Work out the finished part from the listing and answer in its coordinate system (mm). A direction names the side the tool comes from. Give positions to 0.01 mm unless a question says otherwise; leave off trailing zeros. Order: outer loops, then holes, each group sorted by start corner. A loop starts at its lowest first (then second) coordinate and runs counter-clockwise, first axis right, second up. Notation, with made-up numbers: (42.5, 66.5) -> (78.5, 66.5) arc R32 ccw to (78.5, 99.5) -> close; hole circle Ø9 at (84.25, 65.5). An arc over 180 degrees is marked (long way). Answer as CSV lines item,"result". Start each with the question number.
1. A cutting plane is placed at C-C (y = -28). Give the vertices of the cut face in (x, z).
2. Flat-ended cylindrical pins translate along their axes: pin 1 (1.9 mm diameter, centred on x = 19, z = 4, fed in from +Y); pin 2 (1.5 mm diameter, centred on x = -9, z = 1, fed in from +Y); pin 3 (1.9 mm diameter, centred on x = 18, z = 2, fed in from +Y); pin 4 (8 mm diameter, centred on x = 8, y = 55, fed in from -Z). Find the tip coordinate at first contact, or state that the pin passes through.
3. For faces 1 (the flat face through (19, -58.928, 3)), 2 (the flat face through (-1, 1, 0)), determine the directions among +Z, -Z, +X, -X, +Y, -Y from which every point of the face is accessible in a straight line to the end or side of a thin tool.
4. For a pull along Y with two mould halves and no side action, classify faces 3 (the flat face through (-19, 65.278, 3)), 4 (the flat face through (-1, 1, 6.35)) as released by +Y, released by -Y, zero draft, split by the parting line, or undercut.
5. A cutting plane is placed at A-A (y = -62). Give the vertices of the cut face in (x, z), then the cut area to 3 significant figures.
6. Find the intervals of material crossed by L1, parallel to Y at x = -23, z = 2.75; L2, parallel to Y at x = 18.5, z = 4.5; L3, parallel to Y at x = 1, z = 5, in increasing order.
7. A cutting plane is placed at B-B (x = 58). Give the vertices of the cut face in (y, z).
from build123d import *

# Parameters (mm, degrees)
F0_W     = 12.7
F0_H     = 6.35
F1_DEPTH = 6.35


with BuildPart() as f1:
    # F0 (on Top) → F1 (new body)
    with BuildSketch(Plane.XY):
        with BuildLine():
            ThreePointArc((0, -74.168), (52.444696, -52.444696), (74.168, 0))
            ThreePointArc((74.168, 0), (-52.444696, 52.444696), (0, -74.168))
        make_face()
        with Locations((-19.05, -62.103)):
            Rectangle(F0_W, F0_H, mode=Mode.SUBTRACT)
        with Locations((19.05, -62.103)):
            Rectangle(F0_W, F0_H, mode=Mode.SUBTRACT)
        with Locations((-19.05, 62.103)):
            Rectangle(F0_W, F0_H, mode=Mode.SUBTRACT)
        with Locations((19.05, 62.103)):
            Rectangle(F0_W, F0_H, mode=Mode.SUBTRACT)
    extrude(amount=F1_DEPTH)


solid = f1.part
Answer sheet:
1,outline,"(-68.68, 0) -> (68.68, 0) -> (68.68, 6.35) -> (-68.68, 6.35) -> close"
2,pin 1,"stops at y = 71.94"
2,pin 2,"stops at y = 73.71"
2,pin 3,"stops at y = 72.18"
2,pin 4,"stops at z = 0"
3,face 1,"+Z, -Z"
3,face 2,"-Z, +X, -X, +Y, -Y"
4,face 3,"undercut"
4,face 4,"zero draft"
5,outline,"(-40.7, 0) -> (-25.4, 0) -> (-25.4, 6.35) -> (-40.7, 6.35) -> close; (-12.7, 0) -> (12.7, 0) -> (12.7, 6.35) -> (-12.7, 6.35) -> close; (25.4, 0) -> (40.7, 0) -> (40.7, 6.35) -> (25.4, 6.35) -> close"
5,area,"356 mm^2"
6,L1,"y = -70.51 to -65.28, -58.93 to 58.93, 65.28 to 70.51"
6,L2,"y = -71.82 to -65.28, -58.93 to 58.93, 65.28 to 71.82"
6,L3,"y = -74.16 to 74.16"
7,outline,"(-46.23, 0) -> (46.23, 0) -> (46.23, 6.35) -> (-46.23, 6.35) -> close"
